For this review, take the finished solid that the model builds, in its own axes (mm). A direction names the side the tool comes from. Round coordinates to 2 decimals unless told otherwise and drop trailing zeros. Write each loop counter-clockwise with the first axis right and the second up, starting at its lowest first coordinate (ties: lowest second). Pieces come first, ordered by that corner, then holes. Notation, with made-up numbers: M 17,10 L 54,10 A12 ccw 54,27 Z; hole C 63,51.5 d5. An arc over 180 degrees is marked long. Answer in a Markdown table with one row per item.
Autodesk Inventor part; units mm, degrees
ref_plane "Work Plane1" through (609.6, 141.732, -393.7) normal (0, 0, -1) x (-1, 0, 0)
ref_plane "Work Plane2" through (0, 141.732, -101.6) normal (0, 0, 1) x (1, 0, 0)
ref_plane "Work Plane3" through (304.8, 0, 0) normal (1, 0, 0) x (0, 0, -1)
sketch "Sketch1" plane through (0, 0, 0) normal (1, 0, 0) x (0, 1, 0)
  line L0 (0, 0) -> (141.732, 0)
  line L1 (141.732, 0) -> (141.732, -495.3)
  line L2 (141.732, -495.3) -> (0, -495.3)
  line L3 (0, -495.3) -> (0, 0)
  dimension "d0" = 495.3
  dimension "d1" = 141.732
extrude "Extrusion1" add sketch "Sketch1" along normal blind 609.6
shell "Shell1" thickness 25.4 removed faces 1 at (203.2, 141.732, -165.1)
sketch "Sketch2" plane through (0, 0, 0) normal (0, 0, 1) x (1, 0, 0)
  line L0 (25.4, 25.4) -> (25.4, 141.732)
  line L1 (584.2, 141.732) -> (584.2, 25.4)
  line L2 (25.4, 25.4) -> (584.2, 25.4)
  line L3 (584.2, 25.4) -> (584.2, 116.332)
  line L4 (584.2, 116.332) -> (25.4, 116.332)
  line L5 (25.4, 116.332) -> (25.4, 25.4)
  point P0 (0, 0)
  dimension "d5" = 90.932
sketch "Sketch4" plane through (0, 0, 0) normal (-1, 0, 0) x (0, 0, 1)
  line L0 (-25.4, 141.732) -> (-25.4, 25.4)
  line L1 (-469.9, 25.4) -> (-469.9, 141.732)
  line L2 (-25.4, 25.4) -> (-469.9, 25.4)
  line L3 (-469.9, 25.4) -> (-469.9, 116.332)
  line L4 (-469.9, 116.332) -> (-25.4, 116.332)
  line L5 (-25.4, 116.332) -> (-25.4, 25.4)
  point P0 (0, 0)
  dimension "d13" = 90.932
extrude "Extrusion6" cut sketch "Sketch4" against normal through all
extrude "Extrusion7" cut sketch "Sketch2" against normal through all
sketch "Sketch9" plane through (609.6, 25.4, -25.4) normal (0, 1, 0) x (1, 0, 0)
  line L0 (-609.6, -25.4) -> (-609.6, 469.9)
  line L1 (-609.6, 469.9) -> (0, 469.9)
  line L2 (0, 469.9) -> (0, -25.4)
  line L3 (-609.6, -25.4) -> (0, -25.4)
  line L4 (-609.6, 444.5) -> (-584.2, 444.5)
  line L5 (-596.9, 444.5) -> (-596.9, 0)
  line L6 (-609.6, 0) -> (-584.2, 0)
  line L7 (-584.2, 444.5) -> (-584.2, 469.9)
  line L8 (-584.2, 457.2) -> (-25.4, 457.2)
  line L9 (-25.4, 444.5) -> (-25.4, 469.9)
  line L10 (-25.4, 444.5) -> (0, 444.5)
  line L11 (-12.7, 444.5) -> (-12.7, 0)
  line L12 (-25.4, 0) -> (0, 0)
  line L13 (-584.2, -25.4) -> (-584.2, 0)
  line L14 (-584.2, -12.7) -> (-25.4, -12.7)
  line L15 (-25.4, -25.4) -> (-25.4, 0)
  line L16 (-609.6, 444.5) -> (-584.2, 444.5)
  line L17 (-596.9, 444.5) -> (-609.6, 444.5)
  line L18 (-609.6, 0) -> (-596.9, 0)
  line L19 (-609.6, 0) -> (-584.2, 0)
  line L20 (-25.4, 457.2) -> (-25.4, 469.9)
  line L21 (-609.6, 469.9) -> (0, 469.9)
  line L22 (-25.4, 444.5) -> (0, 444.5)
  line L23 (-12.7, 444.5) -> (0, 444.5)
  line L24 (-25.4, 457.2) -> (-25.4, 469.9)
  line L25 (-25.4, 0) -> (0, 0)
  line L26 (-12.7, 0) -> (0, 0)
  line L27 (-25.4, -12.7) -> (-25.4, -25.4)
  line L28 (-25.4, -25.4) -> (-584.2, -25.4)
  line L29 (-584.2, -25.4) -> (-584.2, -12.7)
  line L30 (-609.6, 444.5) -> (-609.6, 0)
  line L31 (-609.6, 469.9) -> (-609.6, -25.4)
  line L32 (-584.2, -25.4) -> (-25.4, -25.4)
  line L33 (-584.2, 469.9) -> (-25.4, 469.9)
  line L34 (-25.4, 469.9) -> (-584.2, 469.9)
  line L35 (0, 444.5) -> (0, 0)
  line L36 (0, 444.5) -> (0, 0)
extrude "Extrusion14" add sketch "Sketch9" along normal blind 12.7 contours L0 L4 L5 L6 | L13 L14 L15 L3 | L0 L1 L7 L4 | L1 L9 L8 L7 | L12 L11 L10 L2 | L1 L2 L10 L9
sketch "Sketch10" plane through (0, 0, -495.3) normal (0, -1, 0) x (1, 0, 0)
  line L0 (25.4, 469.9) -> (25.4, 25.4)
  line L1 (0, 495.3) -> (25.4, 495.3)
  line L2 (25.4, 495.3) -> (25.4, 469.9)
  line L3 (25.4, 469.9) -> (0, 469.9)
  line L4 (0, 469.9) -> (0, 495.3)
  line L5 (25.4, 25.4) -> (0, 25.4)
  line L6 (0, 25.4) -> (0, 0)
  line L7 (0, 0) -> (25.4, 0)
  line L8 (25.4, 0) -> (25.4, 25.4)
  line L9 (609.6, 0) -> (609.6, 495.3)
  line L10 (609.6, 0) -> (584.2, 0)
  line L11 (584.2, 0) -> (584.2, 25.4)
  line L12 (584.2, 25.4) -> (609.6, 25.4)
  line L13 (609.6, 25.4) -> (609.6, 0)
  line L14 (584.2, 469.9) -> (25.4, 469.9)
  line L15 (609.6, 495.3) -> (584.2, 495.3)
  line L16 (584.2, 495.3) -> (584.2, 469.9)
  line L17 (584.2, 469.9) -> (609.6, 469.9)
  line L18 (609.6, 469.9) -> (609.6, 495.3)
  dimension "d48" = 25.4
  dimension "d49" = 25.4
  dimension "d50" = 25.4
  dimension "d51" = 25.4
  dimension "d52" = 25.4
  dimension "d53" = 25.4
  dimension "d54" = 25.4
  dimension "d55" = 25.4
extrude "Extrusion15" add sketch "Sketch10" along normal blind 152.4
sketch "Sketch11" plane through (0, -152.4, -495.3) normal (0, -1, 0) x (1, 0, 0)
  line L0 (609.6, 0) -> (609.6, 25.4)
  line L1 (0, 495.3) -> (609.6, 495.3)
  line L2 (609.6, 495.3) -> (609.6, 0)
  line L3 (609.6, 0) -> (0, 0)
  line L4 (0, 0) -> (0, 495.3)
extrude "Extrusion16" add sketch "Sketch11" along normal blind 25.4
sketch "Sketch12" plane through (25.4, 25.4, -12.7) normal (0, 1, 0) x (1, 0, 0)
  line L0 (185.42, 457.2) -> (185.42, 12.7)
  line L1 (373.38, 457.2) -> (373.38, 12.7)
  line L2 (373.38, 457.2) -> (373.38, 12.7)
  line L3 (185.42, 12.7) -> (185.42, 457.2)
  line L4 (373.38, 457.2) -> (373.38, 469.9)
  line L5 (185.42, 469.9) -> (185.42, 457.2)
  line L6 (185.42, 12.7) -> (185.42, 1.0295)
  line L7 (373.38, 1.0295) -> (373.38, 12.7)
  line L8 (185.42, 469.9) -> (373.38, 469.9)
  line L9 (373.38, 469.9) -> (373.38, 1.0295)
  line L10 (373.38, 1.0295) -> (185.42, 1.0295)
  line L11 (185.42, 1.0295) -> (185.42, 469.9)
  line L12 (558.8, 0) -> (0, 0)
  line L13 (185.42, 469.9) -> (172.72, 469.9)
  line L14 (172.72, 469.9) -> (172.72, 0)
  line L15 (172.72, 0) -> (185.42, 0)
  line L16 (185.42, 0) -> (185.42, 469.9)
  line L17 (373.38, 469.9) -> (386.08, 469.9)
  line L18 (386.08, 469.9) -> (386.08, -5.7755)
  line L19 (386.08, -5.7755) -> (373.38, -5.7755)
  line L20 (373.38, -5.7755) -> (373.38, 469.9)
  dimension "d64" = 12.7
  dimension "d65" = 12.7
extrude "Extrusion17" cut sketch "Sketch12" against normal blind 25.4 contours L5 L8 L4 L1 L7 L10 L6 L0
extrude "Extrusion18" add sketch "Sketch12" along normal blind 12.7 contours L0 L6 L16 L12 L14 L13 L5 | L17 L18 L12 L20 L7 L1 L4 | L12 L18 L19 L20
sketch "Sketch13" plane through (0, -152.4, -495.3) normal (0, 1, 0) x (1, 0, 0)
  line L0 (609.6, -495.3) -> (0, -495.3)
  line L1 (609.6, 0) -> (609.6, -495.3)
  line L2 (0, -495.3) -> (0, 0)
  line L3 (0, 0) -> (609.6, 0)
  line L4 (584.2, -25.4) -> (584.2, -469.9)
  line L5 (584.2, -469.9) -> (25.4, -469.9)
  line L6 (25.4, -469.9) -> (25.4, -25.4)
  line L7 (25.4, -25.4) -> (584.2, -25.4)
  dimension "d68" = 25.4
extrude "Extrusion19" cut sketch "Sketch13" against normal blind 12.7 contours L4 L5 L6 L7
ref_plane "Work Plane1" through (609.6, 141.732, -393.7) normal (0, 0, -1) x (-1, 0, 0)
ref_plane "Work Plane2" through (0, 141.732, -101.6) normal (0, 0, 1) x (1, 0, 0)
sketch "Sketch14" plane through (0, 141.732, -101.6) normal (0, 0, 1) x (1, 0, 0)
  line L0 (584.2, 0) -> (25.4, 0)
  line L1 (16.946, -12.0735) -> (25.4, 0)
  line L2 (25.4, 0) -> (228.6, 0) construction
  line L3 (25.4, 0) -> (-141.0517, 116.5507)
  line L4 (-141.0517, 116.5507) -> (-148.3361, 106.1475)
  line L5 (-148.3361, 106.1475) -> (18.1156, -10.4032)
  line L6 (18.1156, -10.4032) -> (25.4, 0)
  line L7 (25.4, 0) -> (228.6, 0) construction
  point P0 (0, -141.732)
  dimension "d75" = 203.2
  dimension "d76" = 145
  dimension "d77" = 12.7
sketch "Sketch15" plane through (609.6, 141.732, -393.7) normal (0, 0, -1) x (-1, 0, 0)
  line L0 (584.2, 0) -> (750.6517, 116.5507)
  line L1 (757.9361, 106.1475) -> (591.4844, -10.4032)
  line L2 (750.6517, 116.5507) -> (757.9361, 106.1475)
  line L3 (584.2, 0) -> (750.6517, 116.5507)
  line L4 (750.6517, 116.5507) -> (757.9361, 106.1475)
  line L5 (757.9361, 106.1475) -> (591.4844, -10.4032)
  line L6 (591.4844, -10.4032) -> (584.2, 0)
  point P0 (609.6, -141.732)
extrude "Extrusion20" add sketch "Sketch15" along normal mid plane 25.4
extrude "Extrusion21" add sketch "Sketch14" along normal mid plane 25.4
ref_plane "Work Plane3" through (304.8, 0, 0) normal (1, 0, 0) x (0, 0, -1)
sketch "Sketch16" plane through (609.6, 141.732, -406.4) normal (0, 0, -1) x (-1, 0, 0)
  circle A0 centre (749.0923, 107.7069) radius 25.4
  point P0 (609.6, -141.732)
  point P1 (750.6517, 116.5507)
  point P2 (757.9361, 106.1475)
extrude "Extrusion24" add sketch "Sketch16" against normal up to surface (317.5 mm away)
mirror "Mirror2" about plane through (304.8, 0, 0) normal (1, 0, 0) of "Extrusion24", "Extrusion21", "Extrusion20"
sketch "Sketch17" plane through (584.2, 116.332, -469.9) normal (0, 0, 1) x (1, 0, 0)
  line L0 (12.7, -78.232) -> (25.4, -78.232)
  line L1 (25.4, 0) -> (25.4, -78.232)
  line L2 (0, 0) -> (25.4, 0)
  line L3 (0, 0) -> (0, -90.932)
  line L4 (0, -90.932) -> (12.7, -90.932)
  line L5 (12.7, -90.932) -> (12.7, -78.232)
  point P0 (-584.2, -116.332)
extrude "Extrusion25" cut sketch "Sketch17" against normal blind 12.7
sketch "Sketch18" plane through (584.2, 38.1, -482.6) normal (-1, 0, 0) x (0, 0, 1)
  line L0 (0, 0) -> (0, 78.232)
  line L1 (0, 78.232) -> (-12.7, 78.232)
  line L2 (-12.7, 0) -> (-12.7, 78.232)
  line L3 (-12.7, 0) -> (0, 0)
  point P0 (482.6, -38.1)
extrude "Extrusion26" cut sketch "Sketch18" against normal blind 12.7
properties part number "Battery Cart"
Q1. Machinability: for faces 4 (the face through (309, 116.332, -13)), 5 (the face through (402.7, 116.332, -470.3)), 6 (the face through (597, -75, -469.9)), which of the approach directions +Z, -Z, +X, -X, +Y, -Y give a long, thin tool a straight path to every point of the face, cutting with its end or side? Answer none if there is none.
Found:
| item | result |
|---|---|
| face 4 | +Z, -Z |
| face 5 | none |
| face 6 | +X, -X |
Q2. Take a section at D-D (y = 128.5). State the section outline as (x, z) points, then the cut area to 3 significant figures.
Found:
| item | result |
|---|---|
| outline | M 0,-495.3 L 609.6,-495.3 L 609.6,0 L 0,0 Z; hole M 25.4,-469.9 L 584.2,-469.9 L 584.2,-25.4 L 25.4,-25.4 Z |
| area | 53,500 mm² |
Q3. Insertion check: P1, Ø20.5, axis at y = 124, z = -236.5, coming from the -X side; P2, Ø7.5, axis at y = 127.5, z = -156.5, coming from the +X side; P3, Ø12.5, axis at x = 597.5, z = -293.5, coming from the +Y side. Each pin has a flat end and moves straight along its axis. Give the tip position at first contact, or say it passes through.
Found:
| item | result |
|---|---|
| P1 | x = 0 |
| P2 | x = 609.6 |
| P3 | y = 141.73 |
Q4. Mouldability with a two-part tool opening along Y and no side actions: class faces 1 (the face through (-54, 188, -381)), 2 (the face through (13, -75, -469.9)), 3 (the face through (-44.16, 190.44, -393.52)) as +Y half, -Y half, draft (parallel to the pull), parting line (faces both ways), or undercut.
Found:
| item | result |
|---|---|
| face 1 | draft |
| face 2 | undercut |
| face 3 | +Y half |
Q5. Take a section at B-B (x = 70). State the section outline as (y, z) points, then the cut area to 3 significant figures.
Found:
| item | result |
|---|---|
| outline | M -177.8,-495.3 L -152.4,-495.3 L -152.4,-469.9 L -165.1,-469.9 L -165.1,-25.4 L -152.4,-25.4 L -152.4,0 L -177.8,0 Z; M 0,-495.3 L 38.1,-495.3 L 38.1,-482.6 L 25.4,-482.6 L 25.4,-12.7 L 38.1,-12.7 L 38.1,0 L 0,0 Z; M 116.33,-495.3 L 141.73,-495.3 L 141.73,-469.9 L 116.33,-469.9 Z; M 116.33,-25.4 L 141.73,-25.4 L 141.73,0 L 116.33,0 Z |
| area | 21,100 mm² |
Q6. Take a section at A-A (y = 78). State the section outline as (x, z) points, then the cut area to 3 significant figures.
Found:
| item | result |
|---|---|
| outline | M 0,-495.3 L 25.4,-495.3 L 25.4,-469.9 L 0,-469.9 Z; M 0,-25.4 L 25.4,-25.4 L 25.4,0 L 0,0 Z; M 584.2,-25.4 L 609.6,-25.4 L 609.6,0 L 584.2,0 Z; M 596.9,-495.3 L 609.6,-495.3 L 609.6,-482.6 L 596.9,-482.6 Z |
| area | 2,100 mm² |
Q7. Take a section at C-C (z = -346). State how many separate pieces and enclosed holes the cut face has, then the cut area to 3 significant figures.
Found:
| item | result |
|---|---|
| separate pieces | 7 |
| enclosed holes | 0 |
| area | 25,100 mm² |
Q8. For probe 1 along Y at (x, z) = (514.5, -21); probe 2 along X at (y, z) = (35.5, -315.5); probe 3 along Y at (x, z) = (120, -51.5), list the stretches that pass through material, from the lowest coordinate up.
Found:
| item | result |
|---|---|
| probe 1 | -177.8 to -152.4, 0 to 25.4, 116.33 to 141.73 |
| probe 2 | 0 to 12.7, 198.12 to 210.82, 398.78 to 411.48, 596.9 to 609.6 |
| probe 3 | -177.8 to -165.1, 0 to 25.4 |
